Model file for the job. Use its own axes, mm. Coordinates: 2 decimals unless noted, no trailing zeros. Write each loop counter-clockwise with the first axis right and the second up, starting at its lowest first coordinate (ties: lowest second). Pieces come first, ordered by that corner, then holes. Notation, with made-up numbers: M -21,-27 L 23,-27 A15 ccw 23,-2 Z; hole C 32.25,-29 d5. An arc over 180 degrees is marked long. Put each result on its own line as item: value. Start each with the question number.
Q1. Cut at B-B (x = 22.5). Write the cut outline in (y, z).
Q2. Cut at A-A (z = 127). Write the cut outline in (x, y) (3 decimals).
Q3. Drill centre lines: line 1 along X through (y, z) = (3.4, 129) (3 decimals); line 2 along X through (y, z) = (3.05, 90) (3 decimals); line 3 along Z through (x, y) = (13, 3.75). Where is each one in solid material? Low to high.
Q4. Cut at C-C (z = 13.5). Write the cut outline in (x, y) (3 decimals).
Q5. Drop flat-ended pins along their axis: pin 1 (0.8 mm diameter, centred on y = 3.5, z = 70.5, fed in from +X); pin 2 (0.5 mm diameter, centred on x = 3.5, y = 3.5, fed in from +Z); pin 3 (0.5 mm diameter, centred on y = 3.5, z = 11.5, fed in from -X); pin 4 (2 mm diameter, centred on y = 2, z = 113.5, fed in from -X). Give the stop position or say it passes through.
```python
from build123d import *

# Parameters (mm, degrees)
ESBO_O1_W             = 18
ESBO_O1_H             = 25
RVORE_DEPTH           = 4
ESBO_O2_W             = 5.1
ESBO_O2_H             = 77.5
ENCAIXE_DEPTH         = 5
FILETE2_R             = 1
FILETE3_R             = 1
FILETE4_R             = 1
FILETE5_R             = 1
FILETE6_R             = 1
FILETE7_R             = 1
FILETE8_R             = 1.5
FILETE9_R             = 1.5
FILETE10_R            = 1.5
FILETE11_R            = 1.5
FILETE12_R            = 2
FILETE13_R            = 2
FILETE14_R            = 2
FILETE15_R            = 2
FILETE16_R            = 1.5
FILETE17_R            = 1.5
CORTES_DO_LED_DEPTH   = 10
ESBO_O6_W             = 16.486143217
ESBO_O6_H             = 1.199999983
ESBO_O6_W_2           = 1.200000015
ESBO_O6_H_2           = 34.2751352
ESBO_O6_W_3           = 5.711274815
ESBO_O6_H_3           = 1.2
ESBO_O6_W_4           = 1.2
ESBO_O6_H_4           = 71.40185633
CORTE_EXTRUS_O4_DEPTH = 1
FILETE18_R            = 1.5


with BuildPart() as part:
    # Esboço1 → rvore (new body)
    with BuildSketch(Plane(origin=(0, 0, 0), x_dir=(1, 0, 0), z_dir=(0, 1, 0))):
        with Locations((0, -127.5)):
            Rectangle(ESBO_O1_W, ESBO_O1_H)
        Polygon((-51.961524227, -115), (-9, -115), (9, -115), (51.961524227, -115), (30.310889132, -77.5), (-30.310889132, -77.5), align=None)
        Polygon((-8.660254038, -40), (-30.310889132, -77.5), (30.310889132, -77.5), (8.660254038, -40), align=None)
        Polygon((-17.320508076, -40), (-8.660254038, -40), (0, -25), (8.660254038, -40), (17.320508076, -40), (0, -10), align=None)
        Polygon((8.660254038, -40), (30.310889132, -77.5), (38.97114317, -77.5), (17.320508076, -40), align=None)
        Polygon((0, -25), (-8.660254038, -40), (8.660254038, -40), align=None)
        Polygon((-38.97114317, -77.5), (-30.310889132, -77.5), (-8.660254038, -40), (-17.320508076, -40), align=None)
        Polygon((-25.980762114, -40), (-17.320508076, -40), (0, -10), (17.320508076, -40), (25.980762114, -40), (7.216878365, -7.5), (-7.216878365, -7.5), align=None)
        Polygon((0, 5), (-7.216878365, -7.5), (7.216878365, -7.5), align=None)
        Polygon((-12.990381057, -7.5), (-7.216878365, -7.5), (0, 5), (7.216878365, -7.5), (12.990381057, -7.5), (0, 15), align=None)
    extrude(amount=RVORE_DEPTH)

    # Esboço2 → Encaixe (cut)
    with BuildSketch(Plane(origin=(0, 4, 0), x_dir=(1, 0, 0), z_dir=(0, 1, 0))):
        with Locations((0, -101.25)):
            Rectangle(ESBO_O2_W, ESBO_O2_H)
    extrude(amount=-ENCAIXE_DEPTH, mode=Mode.SUBTRACT)

    # Filete2
    filete2_edges = [part.edges().sort_by_distance(p)[0] for p in [
        (12.990381057, 2, 7.5),
    ]]
    fillet(filete2_edges, radius=FILETE2_R)

    # Filete3
    filete3_edges = [part.edges().sort_by_distance(p)[0] for p in [
        (-12.990381057, 2, 7.5),
    ]]
    fillet(filete3_edges, radius=FILETE3_R)

    # Filete4
    filete4_edges = [part.edges().sort_by_distance(p)[0] for p in [
        (-7.216878365, 2, 7.5),
    ]]
    fillet(filete4_edges, radius=FILETE4_R)

    # Filete5
    filete5_edges = [part.edges().sort_by_distance(p)[0] for p in [
        (7.216878365, 2, 7.5),
    ]]
    fillet(filete5_edges, radius=FILETE5_R)

    # Filete6
    filete6_edges = [part.edges().sort_by_distance(p)[0] for p in [
        (25.980762114, 2, 40),
    ]]
    fillet(filete6_edges, radius=FILETE6_R)

    # Filete7
    filete7_edges = [part.edges().sort_by_distance(p)[0] for p in [
        (-25.980762114, 2, 40),
    ]]
    fillet(filete7_edges, radius=FILETE7_R)

    # Filete8
    filete8_edges = [part.edges().sort_by_distance(p)[0] for p in [
        (17.320508076, 2, 40),
    ]]
    fillet(filete8_edges, radius=FILETE8_R)

    # Filete9
    filete9_edges = [part.edges().sort_by_distance(p)[0] for p in [
        (-17.320508076, 2, 40),
    ]]
    fillet(filete9_edges, radius=FILETE9_R)

    # Filete10
    filete10_edges = [part.edges().sort_by_distance(p)[0] for p in [
        (38.97114317, 2, 77.5),
    ]]
    fillet(filete10_edges, radius=FILETE10_R)

    # Filete11
    filete11_edges = [part.edges().sort_by_distance(p)[0] for p in [
        (-38.97114317, 2, 77.5),
    ]]
    fillet(filete11_edges, radius=FILETE11_R)

    # Filete12
    filete12_edges = [part.edges().sort_by_distance(p)[0] for p in [
        (51.961524227, 2, 115),
    ]]
    fillet(filete12_edges, radius=FILETE12_R)

    # Filete13
    filete13_edges = [part.edges().sort_by_distance(p)[0] for p in [
        (-51.961524227, 2, 115),
    ]]
    fillet(filete13_edges, radius=FILETE13_R)

    # Filete14
    filete14_edges = [part.edges().sort_by_distance(p)[0] for p in [
        (9, 2, 115),
    ]]
    fillet(filete14_edges, radius=FILETE14_R)

    # Filete15
    filete15_edges = [part.edges().sort_by_distance(p)[0] for p in [
        (-9, 2, 115),
    ]]
    fillet(filete15_edges, radius=FILETE15_R)

    # Filete16
    filete16_edges = [part.edges().sort_by_distance(p)[0] for p in [
        (30.310889132, 2, 77.5),
    ]]
    fillet(filete16_edges, radius=FILETE16_R)

    # Filete17
    filete17_edges = [part.edges().sort_by_distance(p)[0] for p in [
        (-30.310889132, 2, 77.5),
    ]]
    fillet(filete17_edges, radius=FILETE17_R)

    # Esboço5 → Cortes do Led (cut)
    with BuildSketch(Plane(origin=(0, 4, 0), x_dir=(1, 0, 0), z_dir=(0, 1, 0))):
        Polygon((42.319473419, -98.299478112), (39.519473419, -93.449735851), (36.921397208, -94.949735851), (39.721397208, -99.799478112), align=None)
        Polygon((29.544605065, -61.172757061), (26.744605065, -56.3230148), (24.146528853, -57.8230148), (26.946528853, -62.672757061), align=None)
        Polygon((17.99973671, -26.176458504), (15.19973671, -21.326716243), (12.601660498, -22.826716243), (15.401660498, -27.676458504), align=None)
        Polygon((7.461855653, 2.07568689), (4.661855653, 6.925429151), (2.063779442, 5.425429151), (4.863779442, 0.57568689), align=None)
        Polygon((-7.461855653, 2.07568689), (-4.661855653, 6.925429151), (-2.063779442, 5.425429151), (-4.863779442, 0.57568689), align=None)
        Polygon((-17.99973671, -26.176458504), (-15.19973671, -21.326716243), (-12.601660498, -22.826716243), (-15.401660498, -27.676458504), align=None)
        Polygon((-29.544605065, -61.172757061), (-26.744605065, -56.3230148), (-24.146528853, -57.8230148), (-26.946528853, -62.672757061), align=None)
        Polygon((-42.319473419, -98.299478112), (-39.519473419, -93.449735851), (-36.921397208, -94.949735851), (-39.721397208, -99.799478112), align=None)
    extrude(amount=-CORTES_DO_LED_DEPTH, mode=Mode.SUBTRACT)

    # Esboço6 → Corte-extrusão4 (cut)
    with BuildSketch(Plane(origin=(0, 4, 0), x_dir=(1, 0, 0), z_dir=(0, 1, 0))):
        with BuildLine():
            Line((26.861143157, -102.524864809), (26.861143157, -103.724864792))
            ThreePointArc((26.861143157, -103.724864792), (28.465821261, -103.513604912), (29.96114317, -102.894222224))
            Line((29.96114317, -102.894222224), (29.36114317, -101.854991739))
            ThreePointArc((29.36114317, -101.854991739), (28.155238411, -102.354493936), (26.861143157, -102.524864809))
        make_face()
        with Locations((18.618071549, -103.124864801)):
            Rectangle(ESBO_O6_W, ESBO_O6_H)
        Polygon((38.021397208, -96.854991739), (29.36114317, -101.854991739), (29.96114317, -102.894222224), (38.621397208, -97.894222224), align=None)
        with BuildLine():
            ThreePointArc((10.37499994, -103.724864792), (8.960786372, -104.310651232), (8.375000015, -105.7248648))
            Line((8.375000015, -105.7248648), (7.175, -105.7248648))
            ThreePointArc((7.175, -105.7248648), (8.112258246, -103.462123106), (10.37499994, -102.524864809))
            Line((10.37499994, -102.524864809), (10.37499994, -103.724864792))
        make_face()
        with Locations((7.775000008, -122.8624324)):
            Rectangle(ESBO_O6_W_2, ESBO_O6_H_2)
        Polygon((25.246528853, -59.728270689), (16.586274815, -64.728270689), (17.186274815, -65.767501173), (25.846528853, -60.767501173), align=None)
        with BuildLine():
            Line((14.086274815, -66.59814367), (14.086274815, -65.39814367))
            ThreePointArc((14.086274815, -65.39814367), (15.380370041, -65.227772801), (16.586274815, -64.728270689))
            Line((16.586274815, -64.728270689), (17.186274815, -65.767501173))
            ThreePointArc((17.186274815, -65.767501173), (15.690952895, -66.386883793), (14.086274815, -66.59814367))
        make_face()
        with Locations((11.230637408, -65.99814367)):
            Rectangle(ESBO_O6_W_3, ESBO_O6_H_3)
        with BuildLine():
            ThreePointArc((8.375, -66.59814367), (6.960786438, -67.183930107), (6.375, -68.59814367))
            Line((6.375, -68.59814367), (5.175, -68.59814367))
            ThreePointArc((5.175, -68.59814367), (6.1122583, -66.33540197), (8.375, -65.39814367))
            Line((8.375, -65.39814367), (8.375, -66.59814367))
        make_face()
        with Locations((5.775, -104.299071835)):
            Rectangle(ESBO_O6_W_4, ESBO_O6_H_4)
        Polygon((4.375, -30.116722081), (4.375, -31.502362727), (14.301660498, -25.771202616), (13.701660498, -24.731972131), align=None)
        Polygon((3.175, -0.788496095), (3.175, -140), (4.375, -140), (4.375, -31.502362727), (3.909355653, -31.771202616), (3.309355653, -30.731972131), (4.375, -30.116722081), (4.375, -0.788496095), align=None)
        Polygon((3.909355653, -31.771202616), (4.375, -31.502362727), (4.375, -30.116722081), (3.309355653, -30.731972131), align=None)
    extrude(amount=-CORTE_EXTRUS_O4_DEPTH, mode=Mode.SUBTRACT)

    # Filete18
    filete18_edges = [part.edges().sort_by_distance(p)[0] for p in [
        (4.375, 3.5, 31.502362727),
    ]]
    fillet(filete18_edges, radius=FILETE18_R)


solid = part.part
```
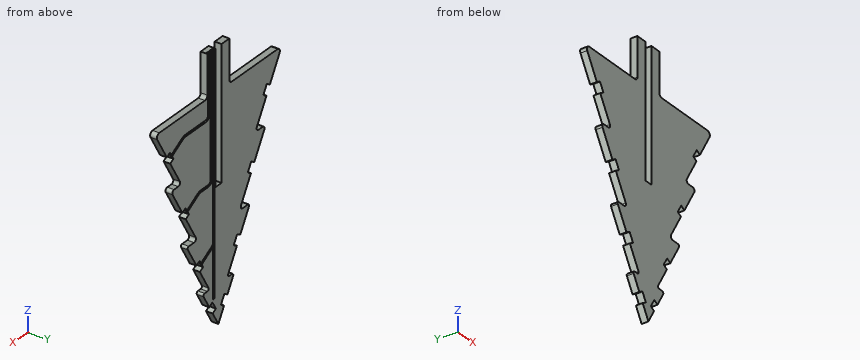
Computed values:
1. outline: M 0,33.97 L 4,33.97 L 4,40 L 0,40 Z; M 0,48.97 L 4,48.97 L 4,61.31 L 3,61.31 L 3,62.7 L 4,62.7 L 4,102.52 L 3,102.52 L 3,103.72 L 4,103.72 L 4,115 L 0,115 Z
2. outline: M -9,0 L -2.55,0 L -2.55,4 L -9,4 Z; M 2.55,0 L 9,0 L 9,4 L 8.375,4 L 8.375,3 L 7.175,3 L 7.175,4 L 6.375,4 L 6.375,3 L 5.175,3 L 5.175,4 L 4.375,4 L 4.375,3 L 3.175,3 L 3.175,4 L 2.55,4 Z
3. line 1: -9 to -2.55, 2.55 to 3.175, 4.375 to 5.175, 6.375 to 7.175, 8.375 to 9
3. line 2: -37.528 to -2.55, 2.55 to 3.175, 4.375 to 5.175, 6.375 to 37.528
3. line 3: 17.52 to 22.6, 23.52 to 25.14, 26.52 to 65.4, 66.6 to 102.52, 103.72 to 115
4. outline: M -10.681,0 L 10.681,0 L 10.681,4 L 4.375,4 L 4.375,3 L 3.175,3 L 3.175,4 L -10.681,4 Z
5. pin 1: x = 35.16
5. pin 2: z = 0.79
5. pin 3: x = -9.67
5. pin 4: x = -50.5
